The drawing under review shows one solid part. Ordinate dimensions are in mm from its lowest x, y, z. A direction names the side the tool comes from. Coordinates: 2 decimals unless noted, no trailing zeros. Write each loop counter-clockwise with the first axis right and the second up, starting at its lowest first coordinate (ties: lowest second). Pieces come first, ordered by that corner, then holes.
1) Insertion check: P1, Ø8, axis at x = 44, z = 28.5, coming from the -Y side; P2, Ø6, axis at y = 5.5, z = 10.5, coming from the -X side; P3, Ø8, axis at x = 56.5, y = 45, coming from the +Z side; P4, Ø16.5, axis at y = 5, z = 12, coming from the +X side. Each pin has a flat end and moves straight along its axis. Give the tip position at first contact, or say it passes through.
2) We need section C-C on x = 62. Write out the cut boundary in (y, z), then the cut area to 3 significant figures.
3) We need section A-A on y = 10. Write out the cut boundary in (x, z), then the cut area to 3 significant figures.
4) To check wall thickness, follow line 1 along Y through (x, z) = (20, 40); line 2 along Z through (x, y) = (14, 52.5); line 3 along Y through (x, z) = (78.5, 18). State the ranges of each line that lie inside material, in increasing order.
5) For the marked faces 1, 2, 3 and 4, list the 3-axis set-ups (+Z, -Z, +X, -X, +Y, -Y) from which the entire face can be reached by the end or side of a thin tool; tool diameter is ignored.
6) We need section B-B on y = 52. Write out the cut boundary in (x, z).
7) Mouldability with a two-part tool opening along X and no side actions: class the marked faces 5, 6 and 7 as pulls with the +X half, pulls with the -X half, needs draft (parallel to the pull), parting line crosses it, or undercut.
8) We need section D-D on z = 9. Write out the cut boundary in (x, y).
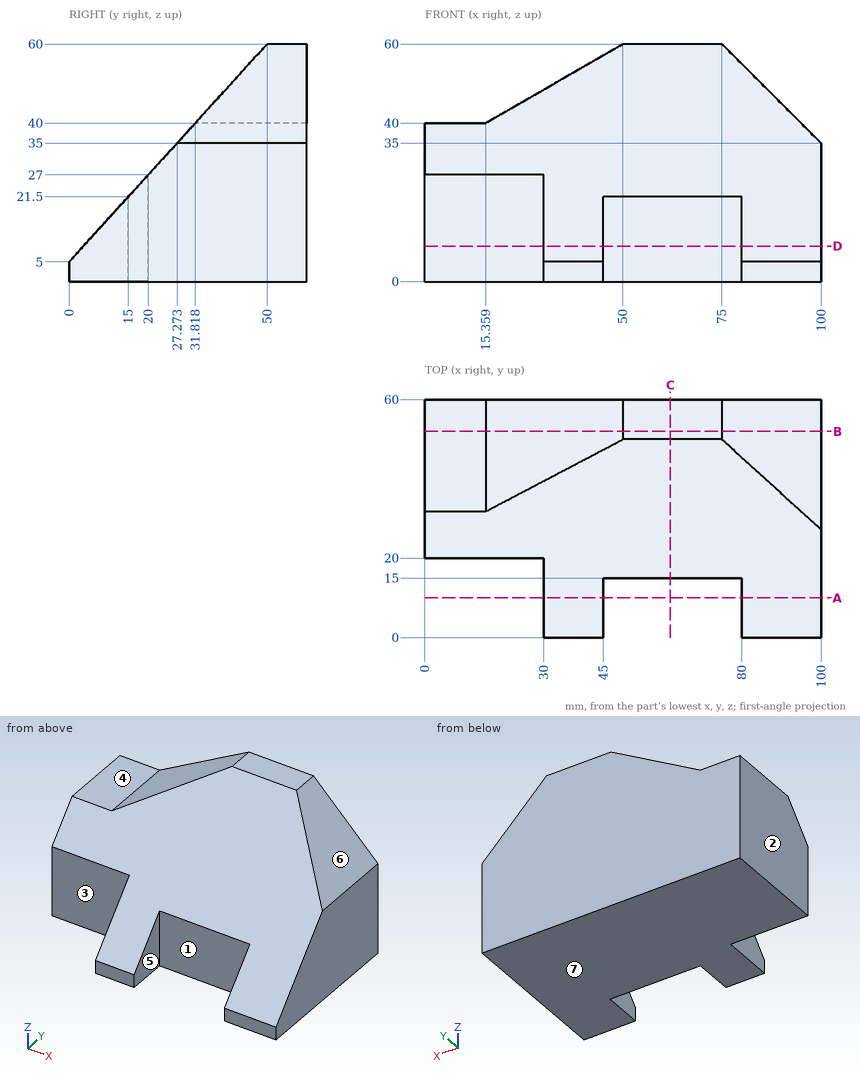
Result:
1. P1: stops at y = 17.73
1. P2: stops at x = 30
1. P3: stops at z = 58.9
1. P4: stops at x = 100
2. outline: (15, 0) - (60, 0) - (60, 60) - (50, 60) - (15, 21.5) - close
2. area: 2,030 mm2
3. outline: (30, 0) - (45, 0) - (45, 16) - (30, 16) - close; (80, 0) - (100, 0) - (100, 16) - (80, 16) - close
3. area: 560 mm2
4. line 1: y = 31.82 to 60
4. line 2: z = 0 to 40
4. line 3: y = 15 to 60
5. face 1: +Z, -Z, -Y
5. face 2: +Z, -Z, -X, +Y, -Y
5. face 3: +Z, -Z, -X, -Y
5. face 4: +Z, -X, +Y, -Y
6. outline: (0, 0) - (100, 0) - (100, 35) - (75, 60) - (50, 60) - (15.36, 40) - (0, 40) - close
7. face 5: undercut
7. face 6: pulls with the +X half
7. face 7: needs draft
8. outline: (0, 20) - (30, 20) - (30, 3.64) - (45, 3.64) - (45, 15) - (80, 15) - (80, 3.64) - (100, 3.64) - (100, 60) - (0, 60) - close
